CAD build for the part. Positions are in the model's coordinates, mm. Face numbers are marked on the shaded views. Give positions to 0.01 mm unless a question says otherwise; leave off trailing zeros. Use one line per item in the form item = value.
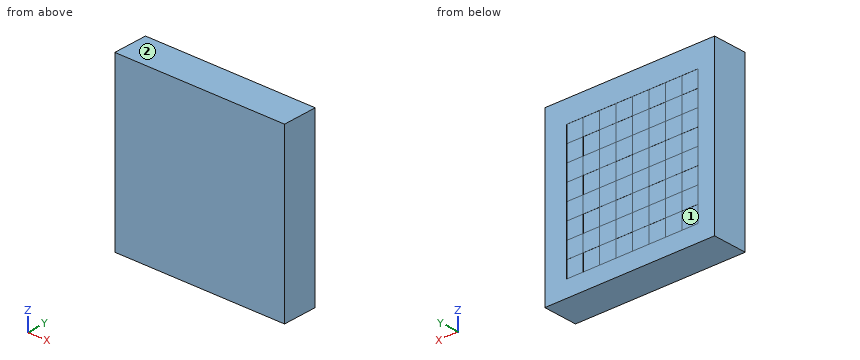
```python
from build123d import *

# Parameters (mm, degrees)
SKETCH1_W                       = 393.7
SKETCH1_H                       = 393.7
BOSS_EXTRUDE1_DEPTH             = 80
ESQUISSE1_W                     = 304.8
ESQUISSE1_H                     = 304.8
ENL_V_MAT_EXTRU_1_DEPTH         = 0.254
ESQUISSE4_W                     = 38.1
ESQUISSE4_H                     = 38.1
ENL_V_MAT_EXTRU_2_DEPTH         = 0.254
R_P_TITION_LIN_AIRE1_COUNT      = 4
R_P_TITION_LIN_AIRE1_PITCH      = 76.2
R_P_TITION_LIN_AIRE1_COUNT_DIR2 = 4
R_P_TITION_LIN_AIRE1_PITCH_DIR2 = 76.2
ESQUISSE5_W                     = 38.1
ESQUISSE5_H                     = 38.1
BOSS_EXTRU_1_DEPTH              = 0.0254
R_P_TITION_LIN_AIRE2_COUNT      = 4
R_P_TITION_LIN_AIRE2_PITCH      = 76.2
R_P_TITION_LIN_AIRE2_COUNT_DIR2 = 4
R_P_TITION_LIN_AIRE2_PITCH_DIR2 = 76.2


with BuildPart() as part:
    # Sketch1 → Boss-Extrude1 (new body)
    with BuildSketch(Plane(origin=(0, 0, 0), x_dir=(1, 0, 0), z_dir=(0, 1, 0))):
        with Locations((196.85, -196.85)):
            Rectangle(SKETCH1_W, SKETCH1_H)
    extrude(amount=BOSS_EXTRUDE1_DEPTH)

    # Esquisse1 → Enlèv. mat.-Extru.1 (cut)
    with BuildSketch(Plane(origin=(0, 80, 0), x_dir=(1, 0, 0), z_dir=(0, 1, 0))):
        with Locations((190.5, -190.5)):
            Rectangle(ESQUISSE1_W, ESQUISSE1_H)
    extrude(amount=-ENL_V_MAT_EXTRU_1_DEPTH, mode=Mode.SUBTRACT)

    # Esquisse4 → Enlèv. mat.-Extru.2 (cut)
    with BuildSketch(Plane(origin=(0, 79.746, 0), x_dir=(1, 0, 0), z_dir=(0, 1, 0))):
        with Locations((57.15, -57.15)):
            Rectangle(ESQUISSE4_W, ESQUISSE4_H)
    enl_v_mat_extru_2 = extrude(amount=-ENL_V_MAT_EXTRU_2_DEPTH, mode=Mode.SUBTRACT)

    # Répétition linéaire1: Enl_v. mat.-Extru.2 4 × 4
    with Locations(*[(i * R_P_TITION_LIN_AIRE1_PITCH, 0, j * R_P_TITION_LIN_AIRE1_PITCH_DIR2) for i in range(R_P_TITION_LIN_AIRE1_COUNT) for j in range(R_P_TITION_LIN_AIRE1_COUNT_DIR2) if (i, j) != (0, 0)]):
        add(enl_v_mat_extru_2, mode=Mode.SUBTRACT)

    # Esquisse5 → Boss.-Extru.1 (add)
    with BuildSketch(Plane(origin=(0, 79.746, 0), x_dir=(1, 0, 0), z_dir=(0, 1, 0))):
        with Locations((95.25, -95.25)):
            Rectangle(ESQUISSE5_W, ESQUISSE5_H)
    boss_extru_1 = extrude(amount=BOSS_EXTRU_1_DEPTH)

    # Répétition linéaire2: Boss.-Extru.1 4 × 4
    with Locations(*[(j * R_P_TITION_LIN_AIRE2_PITCH_DIR2, 0, i * R_P_TITION_LIN_AIRE2_PITCH) for i in range(R_P_TITION_LIN_AIRE2_COUNT) for j in range(R_P_TITION_LIN_AIRE2_COUNT_DIR2) if (i, j) != (0, 0)]):
        add(boss_extru_1)


solid = part.part
```
1. Drill centre lines: line 1 (Y direction, x = 81, z = 244.5); line 2 (Y direction, x = 208, z = 204.5). Where is each one in solid material? Low to high.
Result sheet:
line_1 = 0 to 79.77
line_2 = 0 to 79.49
2. Mould opens along Z. For the marked faces 1 and 2 say: pulls with the +Z half, pulls with the -Z half, needs draft (parallel to the pull), parting line crosses it, or undercut.
Result sheet:
face_1 = undercut
face_2 = pulls with the +Z half
3. Drop flat-ended pins along their axis: P1, Ø11.5, axis at x = 208, z = 50.5, coming from the +Y side; P2, Ø11.5, axis at x = 328.5, z = 164, coming from the +Y side. Give the stop position or say it passes through.
Result sheet:
P1 = 79.49
P2 = 79.77
